The listing builds one solid part. Answer for the finished solid, in the listing's coordinates (mm). Face numbers are marked on the shaded views. A direction names the side the tool comes from. Coordinates: 2 decimals unless noted, no trailing zeros. Order: outer loops, then holes, each group sorted by start corner. A loop starts at its lowest first (then second) coordinate and runs counter-clockwise, first axis right, second up. Notation, with made-up numbers: (-7.75, -19) -> (48.25, -19) arc R25 ccw to (48.25, 0) -> close; hole circle Ø4 at (77.5, 74). An arc over 180 degrees is marked (long way). Answer in a Markdown table with one row per item. Add a question column.
```python
from build123d import *

# Parameters (mm, degrees)
CYLINDER041_R               = 5.35
CYLINDER041_DEPTH           = 12
CYLINDER043_R               = 13
CYLINDER043_DEPTH           = 5
CYLINDER042_R               = 16
CYLINDER042_DEPTH           = 8
CHAMFER003068012002092_SIZE = 0.4


with BuildPart() as cylinder041:
    # Cylinder041 → Cylinder041 (new body)
    with BuildSketch(Plane.XY.offset(-7)):
        Circle(CYLINDER041_R)
    extrude(amount=CYLINDER041_DEPTH)


with BuildPart() as cylinder043:
    # Cylinder043 → Cylinder043 (new body)
    with BuildSketch(Plane.XY.offset(-7)):
        Circle(CYLINDER043_R)
    extrude(amount=CYLINDER043_DEPTH)


with BuildPart() as bearing_remover_top:
    # Cylinder042 → Cylinder042 (new body)
    with BuildSketch(Plane.XY.offset(-10)):
        Circle(CYLINDER042_R)
    extrude(amount=CYLINDER042_DEPTH)

    # Cut001043: cut Cylinder043
    add(cylinder043.part, mode=Mode.SUBTRACT)

    # Fusion001002012037: union Cylinder041
    add(cylinder041.part)

    # Chamfer003068012002092
    chamfer003068012002092_edges = [bearing_remover_top.edges().sort_by_distance(p)[0] for p in [
        (-16, 0, -2),
        (-16, 0, -10),
        (-13, 0, -2),
        (-5.35, 0, 5),
    ]]
    chamfer(chamfer003068012002092_edges, length=CHAMFER003068012002092_SIZE)


solid = bearing_remover_top.part
```
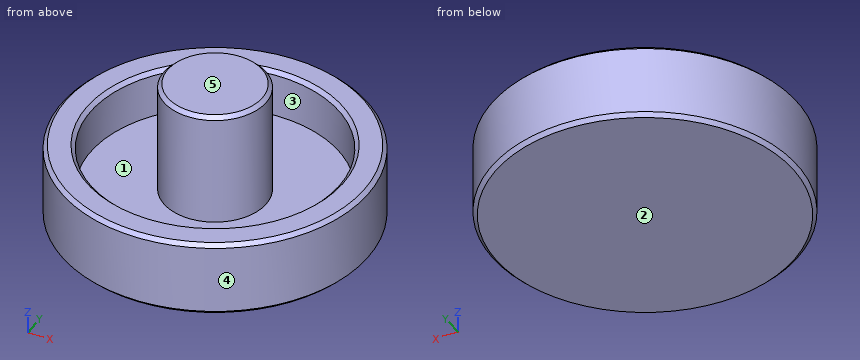
Q1. A cutting plane is placed at D-D (z = -0.5). Determine the outline of the cut face in (x, y).
Q2. A cutting plane is placed at B-B (x = 0). Determine the outline of the cut face in (y, z).
Q3. A cutting plane is placed at A-A (z = -6.25). Determine the outline of the cut face in (x, y).
Q4. Straight lines are drawn through the part: line 1 (Y direction, x = 0, z = -4.45); line 2 (Y direction, x = 2, z = -6.75); line 3 (Z direction, x = -8.5, y = -9.5). For each, find the intervals that lie inside material, in ascending order.
Q5. Given pin 1 (5 mm diameter, centred on x = 6.5, z = -8, fed in from +Y); pin 2 (4 mm diameter, centred on x = 7.5, z = -0.5, fed in from -Y); pin 3 (1.5 mm diameter, centred on x = -8, y = 11, fed in from +Z); pin 4 (13 mm diameter, centred on x = -4.5, y = -5, fed in from +Z), each flat-ended and moving along its own axis, determine where each tip first touches the part or whether it passes through.
Q6. For the marked faces 1 and 2, determine the directions among +Z, -Z, +X, -X, +Y, -Y from which every point of the face is accessible in a straight line to the end or side of a thin tool.
Q7. Determine the mould class of the marked faces 3, 4 and 5 for opening direction X: +X half, -X half, draft (parallel to the pull), parting line (faces both ways), or undercut.
Returned:
| question | item | result |
|---|---|---|
| 1 | outline | circle Ø10.7 at (0, 0) |
| 2 | outline | (-16, -9.6) -> (-15.6, -10) -> (15.6, -10) -> (16, -9.6) -> (16, -2.4) -> (15.6, -2) -> (13.4, -2) -> (13, -2.4) -> (13, -7) -> (5.35, -7) -> (5.35, 4.6) -> (4.95, 5) -> (-4.95, 5) -> (-5.35, 4.6) -> (-5.35, -7) -> (-13, -7) -> (-13, -2.4) -> (-13.4, -2) -> (-15.6, -2) -> (-16, -2.4) -> close |
| 3 | outline | circle Ø32 at (0, 0); circle Ø10.7 at (0, 0); hole circle Ø26 at (0, 0) |
| 4 | line 1 | y = -16 to -13, -5.35 to 5.35, 13 to 16 |
| 4 | line 2 | y = -15.87 to -12.85, -4.96 to 4.96, 12.85 to 15.87 |
| 4 | line 3 | z = -10 to -7 |
| 5 | pin 1 | stops at y = 15.49 |
| 5 | pin 2 | stops at y = -14.46 |
| 5 | pin 3 | stops at z = -2 |
| 5 | pin 4 | stops at z = 5 |
| 6 | face 1 | +Z |
| 6 | face 2 | -Z, +X, -X, +Y, -Y |
| 7 | face 3 | undercut |
| 7 | face 4 | parting line |
| 7 | face 5 | draft |
